```python
from build123d import *

# Parameters (mm, degrees)
F0_R      = 30.329885
F1_DEPTH  = 49.022
F2_R      = 19.689856
F3_DEPTH  = 80.01
F4_R      = 6.735559
F4_R_2    = 6.872412
F5_DEPTH  = 44.196
F3_FACE_R = 19.689856
F6_DEPTH  = 6.604


with BuildPart() as f1:
    # F0 (on Top) → F1 (new body)
    with BuildSketch(Plane.XY):
        Circle(F0_R)
    extrude(amount=F1_DEPTH)

    # F2 (on Top) → F3 (join)
    with BuildSketch(Plane.XY):
        Circle(F2_R)
    extrude(amount=F3_DEPTH)

    # F4 (on Front) → F5 (join)
    with BuildSketch(Plane.XZ):
        with Locations((15.128103, 31.364992)):
            Circle(F4_R)
        with Locations((-10.947968, 32.559317)):
            Circle(F4_R_2)
    extrude(amount=-F5_DEPTH)

    # F3_face (on face) → F6 (join)
    with BuildSketch(Plane.XY.offset(80.01)):
        Circle(F3_FACE_R)
    extrude(amount=-F6_DEPTH)


solid = f1.part
```
Check sheet for the modelled part. Datum: model origin and axes. Units: mm. A direction names the side the tool comes from. Give positions to 0.01 mm unless a question says otherwise; leave off trailing zeros. Order: outer loops, then holes, each group sorted by start corner. A loop starts at its lowest first (then second) coordinate and runs counter-clockwise, first axis right, second up. Notation, with made-up numbers: (63.5, -8.75) -> (108.5, -8.75) arc R19 ccw to (108.5, 22.25) -> close; hole circle Ø1 at (69.25, 34). An arc over 180 degrees is marked (long way). Use CSV: the item, a comma, the result in double quotes. Start each with the question number.
1) Sectioned sample at D-D, the plane x = 16.5. Record the boundary of the cut face in (y, z), plus the area to 3 significant figures.
2) Sectioned sample at A-A, the plane x = 0. Record the boundary of the cut face in (y, z).
3) Mould release check, pull along X, two halves, no side actions. Record for faces 1 (the face through (-17.814, 36.406, 32.861)), 2 (the face through (18.78, 5.91, 64.3)), 3 (the face through (15, 44.196, 31)): released by +X, released by -X, zero draft, split by the parting line, or undercut.
4) Material ranges on line 1 (Z direction, x = -1, y = 22.5); line 2 (Y direction, x = -6, z = 64); line 3 (Y direction, x = -23.5, z = 48.5), recorded low to high. Write a range as from..to.
5) Set-up check for faces 4 (the face through (20, 0, 49.022)), 5 (the face through (21.55, 35.02, 33.39)), 6 (the face through (-11, 44.196, 33)): record each of +Z, -Z, +X, -X, +Y, -Y from which the full face is reachable in a straight line by a thin tool's end or side.
6) Sectioned sample at C-C, the plane z = 70. Record the boundary of the cut face in (x, y).
7) Go/stop test with flat-tipped pins: P1, Ø6, axis at y = 16, z = 58, coming from the -X side; P2, Ø10, axis at y = 2.5, z = 35.5, coming from the -X side; P3, Ø12, axis at y = 22, z = 18, coming from the +X side; P4, Ø1.5, axis at x = 4, z = 41, coming from the -Y side. Record where each tip stops, or that it passes through.
Recorded:
1,outline,"(-25.45, 0) -> (25.45, 0) -> (25.45, 24.77) -> (44.2, 24.77) -> (44.2, 37.96) -> (25.45, 37.96) -> (25.45, 49.02) -> (10.74, 49.02) -> (10.74, 80.01) -> (-10.74, 80.01) -> (-10.74, 49.02) -> (-25.45, 49.02) -> close"
1,area,"3,410 mm2"
2,outline,"(-30.33, 0) -> (30.33, 0) -> (30.33, 49.02) -> (19.69, 49.02) -> (19.69, 80.01) -> (-19.69, 80.01) -> (-19.69, 49.02) -> (-30.33, 49.02) -> close"
3,face 1,"undercut"
3,face 2,"split by the parting line"
3,face 3,"zero draft"
4,line 1,"0..49.02"
4,line 2,"-18.75..18.75"
4,line 3,"-19.17..19.17"
5,face 4,"+Z"
5,face 5,"+Y"
5,face 6,"+Z, -Z, +X, -X, +Y"
6,outline,"circle Ø39.38 at (0, 0)"
7,P1,"x = -14.79"
7,P2,"x = -30.33"
7,P3,"x = 25.77"
7,P4,"y = -30.16"
